For this review, take the finished solid that the model builds, in its own axes (mm). A direction names the side the tool comes from. Coordinates: 2 decimals unless noted, no trailing zeros. Order: outer loops, then holes, each group sorted by start corner. A loop starts at its lowest first (then second) coordinate and runs counter-clockwise, first axis right, second up. Notation, with made-up numbers: (25.25, -18) - (68.25, -18) arc R24 ccw to (68.25, 12) - close; hole circle Ø9 at (79, -25.75). An arc over 180 degrees is marked (long way). One line per item, written item: value. Start each with the question number.
(1) Clearance check with flat-ended pins moving along their axes: pin 1 (5 mm diameter, centred on x = 13, y = 37.5, fed in from +Z); pin 2 (1.5 mm diameter, centred on x = -10, y = 30, fed in from -Z); pin 3 (4 mm diameter, centred on x = 1, y = 49.5, fed in from -Z); pin 4 (9 mm diameter, centred on y = 42.5, z = 15.5, fed in from -X). State where each tip first meets the part, or that it passes through.
(2) Consider section B-B on x = 0. Write out the cut boundary in (y, z), then the cut area to 3 significant figures.
(3) Consider section D-D on y = 33.5. Write out the cut boundary in (x, z).
(4) For faces 5 (the flat face through (12, 38, 8)), 6 (the cylindrical face through (9.515, 43.945, 4.583)), 7 (the flat face through (-12, 40, 8)), list the 3-axis set-ups (+Z, -Z, +X, -X, +Y, -Y) from which the entire face can be reached by the end or side of a thin tool; tool diameter is ignored.
(5) Mouldability with a two-part tool opening along X and no side actions: class faces 1 (the cylindrical face through (-10.16, 48.76, 3.94)), 2 (the flat face through (7, 39, 14)), 3 (the flat face through (-3, 55, 8)), 4 (the cylindrical face through (-7.57, 52.85, 8.6)) as released by +X, released by -X, zero draft, split by the parting line, or undercut.
(6) Consider section C-C on y = 40. Write out the cut boundary in (x, z), then the cut area to 3 significant figures.
(7) To check wall thickness, follow line 1 along X through (y, z) = (30.5, 1.5); line 2 along X through (y, z) = (40, 16); line 3 along X through (y, z) = (40, 7.25). State the ranges of each line that lie inside material, in increasing order.
(8) Consider section A-A on z = 2.5. Write out the cut boundary in (x, y).
```python
from build123d import *

# Parameters (mm, degrees)
SKETCH1_R          = 1.25
MAIN_DEPTH         = 20
SKETCH2_R          = 10.3
CENTRALHOLE_DEPTH  = 12
SKETCH5_R          = 2.75
SKETCH5_W          = 8
SKETCH5_H          = 30
CUT_EXTRUDE3_DEPTH = 12
FILLET1_R          = 2
SKETCH6_W          = 30
SKETCH6_H          = 30
CUT_EXTRUDE4_DEPTH = 21.0000001


with BuildPart() as part:
    # Sketch1 → Main (new body)
    with BuildSketch(Plane.XY):
        Polygon((-15, -15), (5, -15), (15, -5), (15, 15), (-15, 15), align=None)
        with Locations((-10, 10)):
            Circle(SKETCH1_R, mode=Mode.SUBTRACT)
        with Locations((10, 10)):
            Circle(SKETCH1_R, mode=Mode.SUBTRACT)
        with Locations((-10, -10)):
            Circle(SKETCH1_R, mode=Mode.SUBTRACT)
    extrude(amount=MAIN_DEPTH)

    # Sketch2 → CentralHole (cut)
    with BuildSketch(Plane.XY):
        Circle(SKETCH2_R)
    extrude(amount=CENTRALHOLE_DEPTH, mode=Mode.SUBTRACT)

    # Sketch5 → Cut-Extrude3 (cut)
    with BuildSketch(Plane.XY.offset(20)):
        Circle(SKETCH5_R)
        with Locations((11, 0)):
            Rectangle(SKETCH5_W, SKETCH5_H)
        with Locations((-11, 0)):
            Rectangle(SKETCH5_W, SKETCH5_H)
    extrude(amount=-CUT_EXTRUDE3_DEPTH, mode=Mode.SUBTRACT)

    # Fillet1
    fillet1_edges = [part.edges().sort_by_distance(p)[0] for p in [
        (-7, 0, 20),
        (7, 1, 20),
        (-7, 11.27789624, 8),
        (-7, -11.27789624, 8),
        (7, 11.27789624, 8),
        (7, -10.27789624, 8),
    ]]
    fillet(fillet1_edges, radius=FILLET1_R)


with BuildPart() as body_2:
    # Mirror1: mirrored copy
    add(part.part.mirror(Plane.ZX.offset(20)))


with BuildPart() as part_1:
    add(part.part)

    # Sketch6 → Cut-Extrude4 (cut, through all)
    with BuildSketch(Plane.XY.offset(20)):
        Rectangle(SKETCH6_W, SKETCH6_H)
    extrude(amount=-CUT_EXTRUDE4_DEPTH, mode=Mode.SUBTRACT)


solid = body_2.part
```
Geometry check:
1. pin 1: stops at z = 8
1. pin 2: passes through
1. pin 3: stops at z = 0
1. pin 4: stops at x = -7
2. outline: (25, 0) - (29.7, 0) - (29.7, 12) - (37.25, 12) - (37.25, 20) - (25, 20) - close; (42.75, 12) - (50.3, 12) - (50.3, 0) - (55, 0) - (55, 20) - (42.75, 20) - close
2. area: 309 mm^2
3. outline: (-15, 0) - (-7.99, 0) - (-7.99, 8.27) arc R2 cw to (-9, 8) - (-15, 8) - close; (-7, 12) - (7, 12) - (7, 18) arc R2 ccw to (5, 20) - (-5, 20) arc R2 ccw to (-7, 18) - close; (7.99, 0) - (15, 0) - (15, 8) - (9, 8) arc R2 cw to (7.99, 8.27) - close
4. face 5: +Z, +X, +Y, -Y
4. face 6: -Z
4. face 7: +Z, -X, +Y, -Y
5. face 1: undercut
5. face 2: released by +X
5. face 3: zero draft
5. face 4: released by -X
6. outline: (-15, 0) - (-10.3, 0) - (-10.3, 8) - (-15, 8) - close; (-7, 12) - (-2.75, 12) - (-2.75, 20) - (-5, 20) arc R2 ccw to (-7, 18) - close; (2.75, 12) - (7, 12) - (7, 18) arc R2 ccw to (5, 20) - (2.75, 20) - close; (10.3, 0) - (15, 0) - (15, 8) - (10.3, 8) - close
6. area: 141 mm^2
7. line 1: x = -15 to -11.15, -8.85 to -3.98, 3.98 to 8.85, 11.15 to 15
7. line 2: x = -7 to -2.75, 2.75 to 7
7. line 3: x = -15 to -10.3, 10.3 to 15
8. outline: (-15, 25) - (15, 25) - (15, 45) - (5, 55) - (-15, 55) - close; hole circle Ø2.5 at (-10, 30); hole circle Ø2.5 at (-10, 50); hole circle Ø20.6 at (0, 40); hole circle Ø2.5 at (10, 30)
